from build123d import *

# Parameters (mm, degrees)
F1_DEPTH = 25
F2_SIZE  = 10
F3_SIZE  = 10


with BuildPart() as f1:
    # F0 (on Top) → F1 (new body)
    with BuildSketch(Plane.XY):
        Polygon((-37.185604, -26.554091), (-1.63635, -47.264697), (36.720452, -32.384023), (49.001347, 6.882481), (25.958571, 40.966337), (-15.056196, 44.201705), (-43.157998, 14.152288), align=None)
    extrude(amount=F1_DEPTH)

    # F2
    f2_edges = [f1.edges().sort_by_distance(p)[0] for p in [
        (-19.410977, -36.909394, 25),
        (5.451187, 42.584021, 25),
        (-29.107097, 29.176996, 25),
        (-40.171801, -6.200901, 25),
        (17.542051, -39.82436, 25),
        (42.8609, -12.750771, 25),
        (37.479959, 23.924409, 25),
    ]]
    chamfer(f2_edges, length=F2_SIZE)

    # F3
    f3_edges = [f1.edges().sort_by_distance(p)[0] for p in [
        (-29.107097, 29.176996, 0),
        (5.451187, 42.584021, 0),
        (-40.171801, -6.200901, 0),
        (-19.410977, -36.909394, 0),
        (17.542051, -39.82436, 0),
        (42.8609, -12.750771, 0),
        (37.479959, 23.924409, 0),
    ]]
    chamfer(f3_edges, length=F3_SIZE)


solid = f1.part
Here's how the part is built. I have some questions about the finished solid (model axes, mm). Give positions to 0.01 mm unless a question says otherwise; leave off trailing zeros. Loops run counter-clockwise (first coordinate to the right, second up) from the corner with the lowest first, then second, coordinate; pieces in that order, holes last. Notation, with made-up numbers: (2.25, 45) -> (53.25, 45) arc R15 ccw to (53.25, 54) -> close; hole circle Ø6 at (-32.5, -27.5). An arc over 180 degrees is marked (long way). Answer as a JSON object with one key per item and string values. Group by question number.
Item 1: Will these pins go through, and if not, where does the flat tip stop? pin 1 (2 mm diameter, centred on y = -5, z = 5.5, fed in from -X); pin 2 (4 mm diameter, centred on y = -16.5, z = 18, fed in from +X); pin 3 (4 mm diameter, centred on y = 5, z = 21, fed in from +X).
Item 2: Imagine slicing it at C-C on y = -10. Write out the boundary of the cut face in (x, z).
Item 3: I need wall thicknesses on L1, parallel to Y at x = -29.5, z = 4.25; L2, parallel to Y at x = -10, z = 23.5; L3, parallel to X at y = -3.5, z = 4. Which ranges of each line are inside material? Lowest first, please.
Item 4: Imagine slicing it at B-B on x = -23. Write out the boundary of the cut face in (y, z), then the cut area to 3 significant figures.
Item 5: Imagine slicing it at D-D on x = 23. Write out the boundary of the cut face in (y, z), then the cut area to 3 significant figures.
Item 6: Imagine slicing it at A-A on z = 11.75. Write out the boundary of the cut face in (x, y).
Answer list:
{
 "1": {"pin 1": "stops at x = -36.82", "pin 2": "stops at x = 40.73", "pin 3": "stops at x = 44.31"},
 "2": {"outline": "(-39.61, 10) -> (-29.51, 0) -> (33.24, 0) -> (43.72, 10) -> (43.72, 15) -> (33.24, 25) -> (-29.51, 25) -> (-39.61, 15) -> close"},
 "3": {"L1": "y = -24.38 to 20.34", "L2": "y = -32.55 to 35.28", "L3": "x = -34.5 to 39.47"},
 "4": {"outline": "(-34.82, 10) -> (-23.25, 0) -> (21.07, 0) -> (35.71, 10) -> (35.71, 15) -> (21.07, 25) -> (-23.25, 25) -> (-34.82, 15) -> close", "area": "1,500 mm2"},
 "5": {"outline": "(-37.71, 10) -> (-26.98, 0) -> (27.49, 0) -> (35.89, 4.7) -> (41.2, 10) -> (41.2, 15) -> (35.89, 20.3) -> (27.49, 25) -> (-26.98, 25) -> (-37.71, 15) -> close", "area": "1,750 mm2"},
 "6": {"outline": "(-43.16, 14.15) -> (-37.19, -26.55) -> (-1.64, -47.26) -> (36.72, -32.38) -> (49, 6.88) -> (25.96, 40.97) -> (-15.06, 44.2) -> close"}
}
